Check sheet for the drawn part. Datum: minimum x, y, z corner. Units: mm. A direction names the side the tool comes from. Coordinates: 2 decimals unless noted, no trailing zeros. Loops run counter-clockwise (first coordinate to the right, second up) from the corner with the lowest first, then second, coordinate; pieces in that order, holes last.
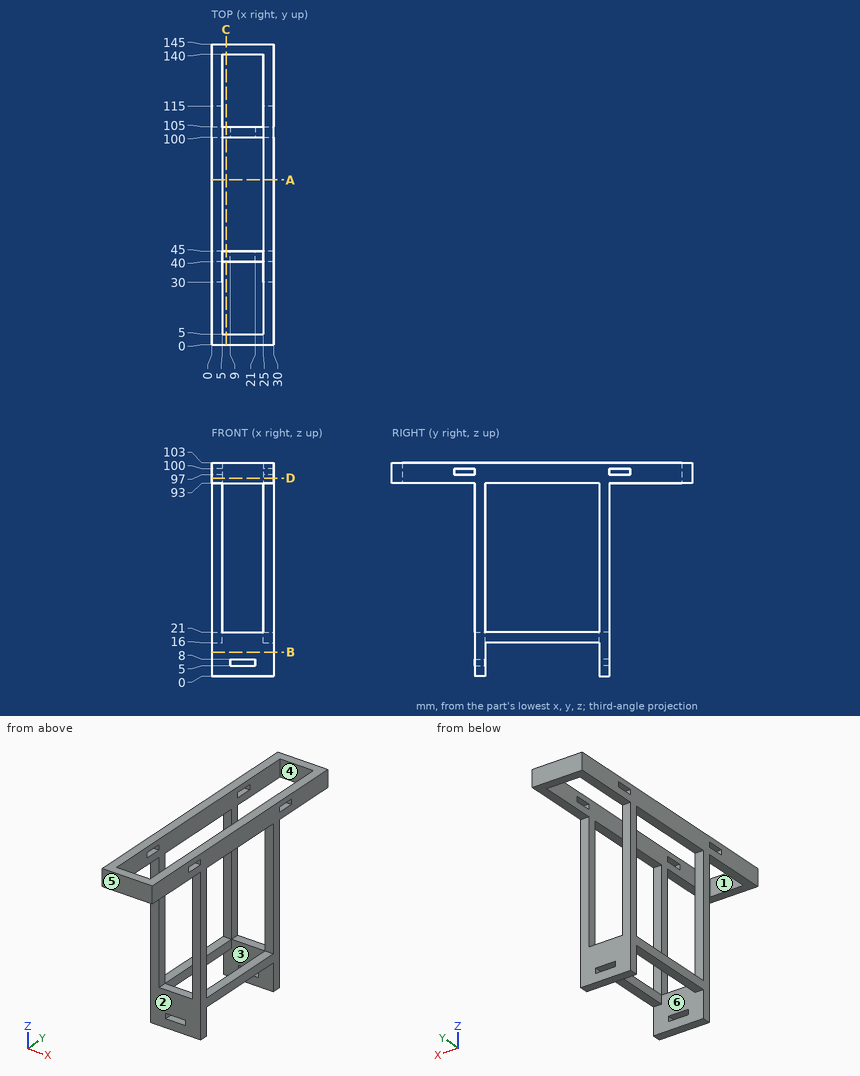
(1) Access from +Z, -Z, +X, -X, +Y, -Y to the whole of each face (thin tool, end or side, straight path). Record for the marked faces 1, 2 and 3.
Findings:
face 1: +Z, -Z
face 2: -Z, +X, -X, -Y
face 3: -Z
(2) Sectioned sample at B-B on z = 11.5. Record the cut outline in (x, y), and give its area (3 significant figures).
Findings:
outline: (0, 40) - (30, 40) - (30, 45) - (0, 45) - close; (0, 100) - (30, 100) - (30, 105) - (0, 105) - close
area: 300 mm2
(3) Gauge pin test, flat ends, axial feed: pin 1 Ø4 at (x, y) = (28, 35) entering from -Z; pin 2 Ø5 at (x, z) = (7, 36) entering from +Y; pin 3 Ø6 at (x, y) = (9, 96) entering from -Z. Record the tip position at first contact, or that the pin passes through.
Findings:
pin 1: stops at z = 93
pin 2: stops at y = 105
pin 3: passes through
(4) Sectioned sample at C-C on x = 7. Record the cut outline in (y, z), and give its area (3 significant figures).
Findings:
outline: (0, 93) - (5, 93) - (5, 103) - (0, 103) - close; (40, 0) - (45, 0) - (45, 21) - (40, 21) - close; (100, 0) - (105, 0) - (105, 21) - (100, 21) - close; (140, 93) - (145, 93) - (145, 103) - (140, 103) - close
area: 310 mm2
(5) Sectioned sample at A-A on y = 79.5. Record the cut outline in (x, z).
Findings:
outline: (0, 16) - (5, 16) - (5, 21) - (0, 21) - close; (0, 93) - (5, 93) - (5, 103) - (0, 103) - close; (25, 16) - (30, 16) - (30, 21) - (25, 21) - close; (25, 93) - (30, 93) - (30, 103) - (25, 103) - close
(6) Sectioned sample at D-D on z = 95.5. Record the cut outline in (x, y).
Findings:
outline: (0, 0) - (30, 0) - (30, 145) - (0, 145) - close; hole (5, 5) - (25, 5) - (25, 140) - (5, 140) - close
(7) Draft check along X on the marked faces 4, 5 and 6. Enter one of: +X half, -X half, draft (parallel to the pull), parting line (faces both ways), or undercut.
Findings:
face 4: undercut
face 5: draft
face 6: undercut
(8) Scan lines: L1, parallel to Y at x = 26.75, z = 48.5; L2, parallel to X at y = 71, z = 98.5; L3, parallel to Z at x = 27, y = 68.5. Record each from-to range of solid material in increasing order.
Findings:
L1: y = 40 to 45, 100 to 105
L2: x = 0 to 5, 25 to 30
L3: z = 16 to 21, 93 to 103
